Could you check a few things on this model? Use its own coordinates, in mm. Give positions to 0.01 mm unless a question says otherwise; leave off trailing zeros. Write each loop counter-clockwise with the first axis right and the second up, starting at its lowest first coordinate (ties: lowest second). Pieces come first, ordered by that corner, then holes. Notation, with made-up numbers: M -30.75,-27.5 L 8.25,-27.5 A26 ccw 8.25,-9.5 Z; hole C -38,42 d6. An arc over 180 degrees is marked long. One line per item, written item: value.
```python
from build123d import *

# Parameters (mm, degrees)
SKETCH_1_R          = 1
SKETCH_1_R_2        = 7.25
EXTRUDE_1_DEPTH     = 5
SKETCH_2_R          = 1.5
CUT_EXTRUDE_1_DEPTH = 10
SKETCH_3_R          = 1.5
CUT_EXTRUDE_2_DEPTH = 10
FILLET_1_R          = 2
CHAMFER_1_SIZE      = 6.5
SKETCH_4_R          = 1
CUT_EXTRUDE_3_DEPTH = 10
SKETCH_6_W          = 10
SKETCH_6_H          = 12
SKETCH_6_R          = 2.5
EXTRUDE_2_DEPTH     = 5
FILLET_2_R          = 1


with BuildPart() as part:
    # 草图1 → 凸台-拉伸1 (new body)
    with BuildSketch(Plane.XY):
        with BuildLine():
            Line((95, -15), (95, 15))
            Line((95, 15), (33, 15))
            ThreePointArc((33, 15), (28.757359313, 16.757359313), (27, 21))
            Line((27, 21), (18, 21))
            Line((18, 21), (12, 27))
            Line((12, 27), (-12, 27))
            Line((-12, 27), (-18, 21))
            Line((-18, 21), (-27, 21))
            ThreePointArc((-27, 21), (-28.757359313, 16.757359313), (-33, 15))
            Line((-33, 15), (-95, 15))
            Line((-95, 15), (-95, -15))
            Line((-95, -15), (-33, -15))
            ThreePointArc((-33, -15), (-28.757359313, -16.757359313), (-27, -21))
            Line((-27, -21), (-18, -21))
            Line((-18, -21), (-12, -27))
            Line((-12, -27), (12, -27))
            Line((12, -27), (18, -21))
            Line((18, -21), (27, -21))
            ThreePointArc((27, -21), (28.757359313, -16.757359313), (33, -15))
            Line((33, -15), (95, -15))
        make_face()
        with Locations((0, 9.5)):
            Circle(SKETCH_1_R, mode=Mode.SUBTRACT)
        Circle(SKETCH_1_R_2, mode=Mode.SUBTRACT)
        with Locations((8.227241336, -4.75)):
            Circle(SKETCH_1_R, mode=Mode.SUBTRACT)
        with Locations((-8.227241336, -4.75)):
            Circle(SKETCH_1_R, mode=Mode.SUBTRACT)
    extrude(amount=EXTRUDE_1_DEPTH)

    # 草图2 → 切除-拉伸1 (cut)
    with BuildSketch(Plane.XY.offset(5)):
        with Locations((7, 23)):
            Circle(SKETCH_2_R)
        with Locations((-7, 23)):
            Circle(SKETCH_2_R)
        with Locations((7, -23)):
            Circle(SKETCH_2_R)
        with Locations((-7, -23)):
            Circle(SKETCH_2_R)
    extrude(amount=-CUT_EXTRUDE_1_DEPTH, mode=Mode.SUBTRACT)

    # 草图3 → 切除-拉伸2 (cut)
    with BuildSketch(Plane.XY.offset(5)):
        with Locations((87.5, 0)):
            Circle(SKETCH_3_R)
        with Locations((72.5, 0)):
            Circle(SKETCH_3_R)
        with Locations((57.5, 0)):
            Circle(SKETCH_3_R)
        with Locations(Location((-57.5, 0, 0), (0, 0, 180))):
            Circle(SKETCH_3_R)
        with Locations(Location((-72.5, 0, 0), (0, 0, 180))):
            Circle(SKETCH_3_R)
        with Locations(Location((-87.5, 0, 0), (0, 0, 180))):
            Circle(SKETCH_3_R)
        with Locations((42.5, 0)):
            Circle(SKETCH_3_R)
        with Locations((27.5, 0)):
            Circle(SKETCH_3_R)
        with Locations(Location((-27.5, 0, 0), (0, 0, 180))):
            Circle(SKETCH_3_R)
        with Locations(Location((-42.5, 0, 0), (0, 0, 180))):
            Circle(SKETCH_3_R)
    extrude(amount=-CUT_EXTRUDE_2_DEPTH, mode=Mode.SUBTRACT)

    # 圆角1
    fillet_1_edges = [part.edges().sort_by_distance(p)[0] for p in [
        (18, -21, 2.5),
        (-18, -21, 2.5),
        (-18, 21, 2.5),
        (18, 21, 2.5),
    ]]
    fillet(fillet_1_edges, radius=FILLET_1_R)

    # 倒角1
    chamfer_1_edges = [part.edges().sort_by_distance(p)[0] for p in [
        (95, 15, 2.5),
        (95, -15, 2.5),
        (-95, -15, 2.5),
        (-95, 15, 2.5),
    ]]
    chamfer(chamfer_1_edges, length=CHAMFER_1_SIZE)

    # 草图4 → 切除-拉伸3 (cut)
    with BuildSketch(Plane.XY.offset(5)):
        with Locations((85, 12.5)):
            Circle(SKETCH_4_R)
        with Locations((85, -12.5)):
            Circle(SKETCH_4_R)
        with Locations(Location((-85, -12.5, 0), (0, 0, 180))):
            Circle(SKETCH_4_R)
        with Locations(Location((-85, 12.5, 0), (0, 0, 180))):
            Circle(SKETCH_4_R)
    extrude(amount=-CUT_EXTRUDE_3_DEPTH, mode=Mode.SUBTRACT)

    # 草图6 → 凸台-拉伸2 (add)
    with BuildSketch(Plane(origin=(0, 0, 0), x_dir=(-1, 0, 0), z_dir=(0, 0, -1))):
        with Locations((39, 21)):
            Rectangle(SKETCH_6_W, SKETCH_6_H)
        with Locations((38.97114317, 22.5)):
            Circle(SKETCH_6_R, mode=Mode.SUBTRACT)
    extrude(amount=-EXTRUDE_2_DEPTH)

    # 圆角2
    fillet_2_edges = [part.edges().sort_by_distance(p)[0] for p in [
        (-44, 15, 2.5),
        (-34, 15, 2.5),
    ]]
    fillet(fillet_2_edges, radius=FILLET_2_R - 0.0001)  # a hair under: the kernel refuses the full size
    fillet_2_2_edges = [part.edges().sort_by_distance(p)[0] for p in [
        (-34, 27, 2.5),
        (-44, 27, 2.5),
    ]]
    fillet(fillet_2_2_edges, radius=FILLET_2_R)


solid = part.part
```
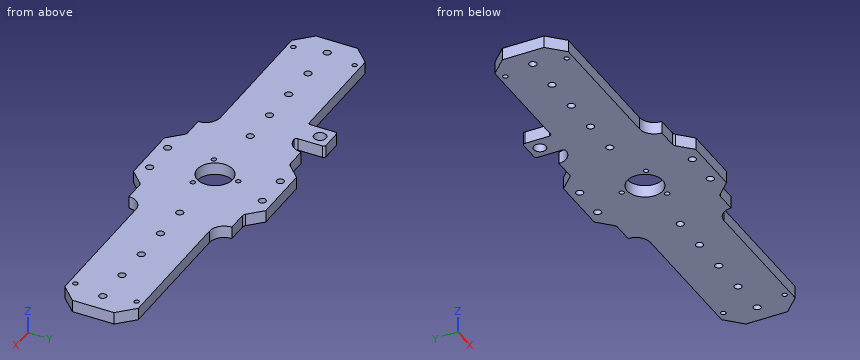
1) Please list where these lines run through material, in increasing order: L1, parallel to Y at x = -85, z = 2.5; L2, parallel to Y at x = -87.5, z = 2.4; L3, parallel to X at y = -12, z = 3.8. Write a range as from..to.
Outcome:
L1: y = -15..-13.5, -11.5..11.5, 13.5..15
L2: y = -15..-1.5, 1.5..15
L3: x = -91.5..-85.87, -84.13..84.13, 85.87..91.5
2) I'm going to push flat-ended pins straight in: pin 1 (1.5 mm diameter, centred on y = -11, z = 4, fed in from +X); pin 2 (1.5 mm diameter, centred on x = 38, z = 3, fed in from +Y); pin 3 (2.5 mm diameter, centred on x = -57.5, y = 0, fed in from -Z); pin 4 (2.5 mm diameter, centred on y = 23, z = 1.5, fed in from -X). Where does each tip first touch, or does it pass through?
Outcome:
pin 1: stops at x = 93.25
pin 2: stops at y = 15
pin 3: passes through
pin 4: stops at x = -44
3) If we section it at C-C, the plane y = -19: Write out the boundary of the cut face in (x, z).
Outcome:
outline: M -27.34,0 L 27.34,0 L 27.34,5 L -27.34,5 Z
4) If we section it at A-A, the plane z = 2: Give the number of separate pieces and of enclosed holes in the cut face, then the cut area to 3 significant figures.
Outcome:
separate pieces: 1
enclosed holes: 23
area: 6,470 mm^2
5) If we section it at B-B, the plane x = -53: Write out the boundary of the cut face in (y, z).
Outcome:
outline: M -15,0 L 15,0 L 15,5 L -15,5 Z
